Check sheet for the drawn part. Datum: minimum x, y, z corner. Units: mm. A direction names the side the tool comes from. Give positions to 0.01 mm unless a question says otherwise; leave off trailing zeros. Write each loop counter-clockwise with the first axis right and the second up, starting at its lowest first coordinate (ties: lowest second). Pieces come first, ordered by that corner, then holes. Notation, with made-up numbers: (50, -12) - (81, -12) arc R15 ccw to (81, 9) - close; hole circle Ø6 at (71.25, 0.25). An arc over 180 degrees is marked (long way). Use a Markdown table: item, result.
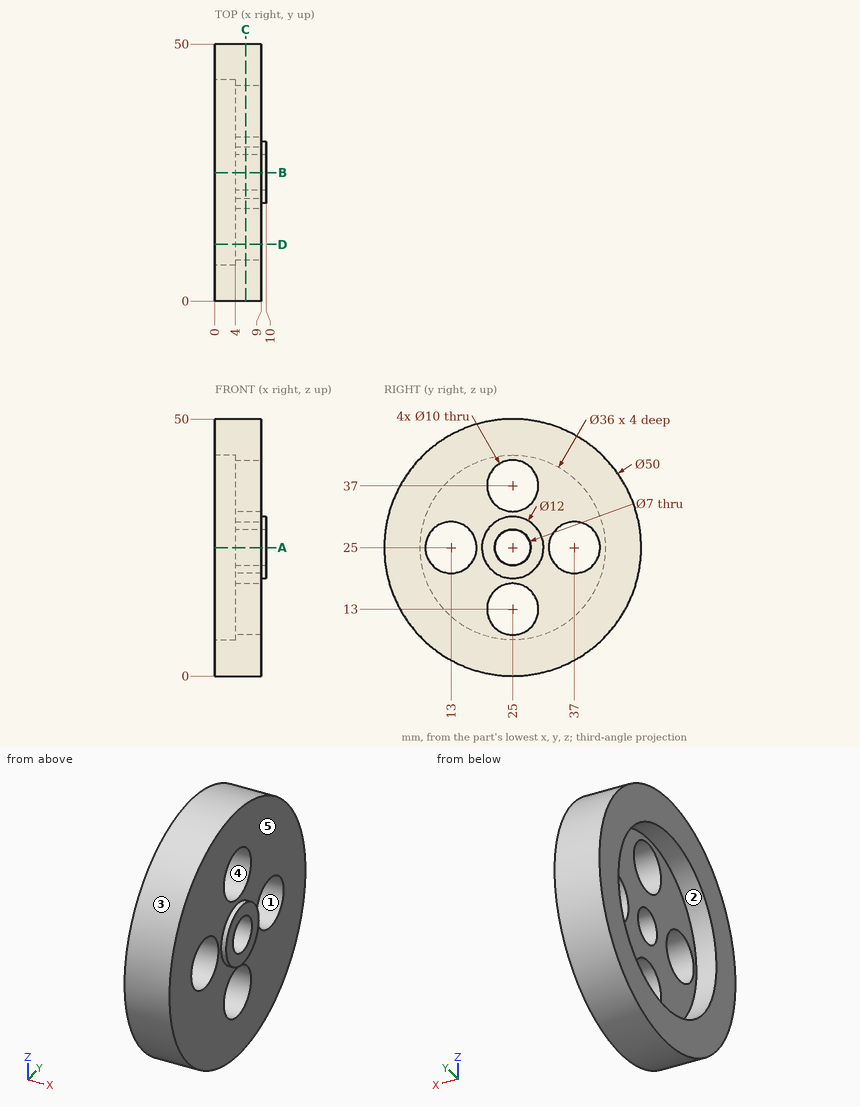
1) Mould release check, pull along Y, two halves, no side actions. Record for the marked faces 3, 4 and 5: pulls with the +Y half, pulls with the -Y half, needs draft (parallel to the pull), parting line crosses it, or undercut.
Working result:
| item | result |
|---|---|
| face 3 | parting line crosses it |
| face 4 | undercut |
| face 5 | needs draft |
2) Section check D-D on y = 11. Record the boundary of the cut face in (x, z).
Working result:
| item | result |
|---|---|
| outline | (0, 4.29) - (9, 4.29) - (9, 20.42) - (4, 20.42) - (4, 13.69) - (0, 13.69) - close; (0, 36.31) - (4, 36.31) - (4, 29.58) - (9, 29.58) - (9, 45.71) - (0, 45.71) - close |
3) Depth check by flat-ended pin: P1, Ø1.5, axis at x = 6.5, y = 37.5, coming from the +Z side; P2, Ø11, axis at y = 25, z = 25, coming from the -X side; P3, Ø8, axis at y = 25, z = 37, coming from the +X side; P4, Ø16, axis at y = 37, z = 25, coming from the -X side. Enter the tip coordinate at first touch or a pass-through.
Working result:
| item | result |
|---|---|
| P1 | stops at z = 47.07 |
| P2 | stops at x = 4 |
| P3 | passes through |
| P4 | stops at x = 0 |
4) Set-up check for the marked faces 1 and 2: record each of +Z, -Z, +X, -X, +Y, -Y from which the full face is reachable in a straight line by a thin tool's end or side.
Working result:
| item | result |
|---|---|
| face 1 | +X, -X |
| face 2 | -X |
5) Section check A-A on z = 25. Record the boundary of the cut face in (x, y).
Working result:
| item | result |
|---|---|
| outline | (0, 0) - (9, 0) - (9, 8) - (4, 8) - (4, 7) - (0, 7) - close; (0, 43) - (4, 43) - (4, 42) - (9, 42) - (9, 50) - (0, 50) - close; (4, 18) - (9, 18) - (9, 19) - (10, 19) - (10, 21.5) - (4, 21.5) - close; (4, 28.5) - (10, 28.5) - (10, 31) - (9, 31) - (9, 32) - (4, 32) - close |
6) Section check C-C on x = 6. Record the boundary of the cut face in (y, z), then the cut area to 3 significant figures.
Working result:
| item | result |
|---|---|
| outline | circle Ø50 at (25, 25); hole circle Ø10 at (13, 25); hole circle Ø10 at (25, 13); hole circle Ø10 at (25, 37); hole circle Ø7 at (25, 25); hole circle Ø10 at (37, 25) |
| area | 1,610 mm² |
7) Material ranges on L1, parallel to Y at x = 2, z = 25; L2, parallel to Z at x = 2.5, y = 24.5 (3 decimals); L3, parallel to Z at x = 8.75, y = 27, recorded low to high. Write a range as from..to.
Working result:
| item | result |
|---|---|
| L1 | y = 0..7, 43..50 |
| L2 | z = 0.005..7.007, 42.993..49.995 |
| L3 | z = 0.08..8.42, 17.58..22.13, 27.87..32.42, 41.58..49.92 |
